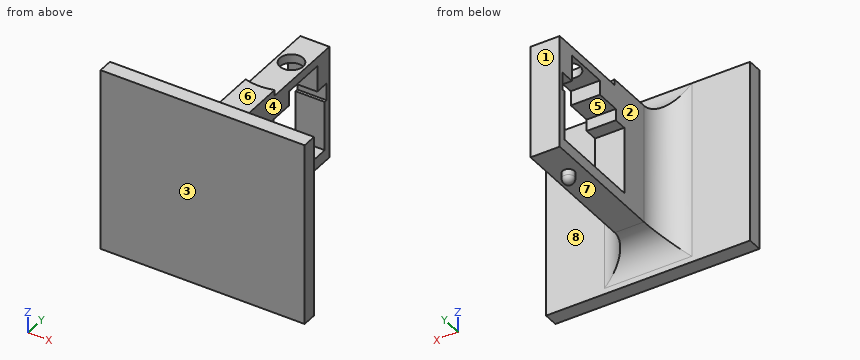
```python
from build123d import *

# Parameters (mm, degrees)
BOSS_EXTRUDE1_DEPTH      = 20
BOSS_EXTRUDE1_DEPTH_BACK = 43
SKETCH1_W                = 70
SKETCH1_H                = 5
BOSS_EXTRUDE2_DEPTH      = 10
BOSS_EXTRUDE2_DEPTH_BACK = 10
SKETCH2_W                = 10
SKETCH2_H                = 55
CUT_EXTRUDE2_DEPTH       = 10
CUT_EXTRUDE2_DEPTH_BACK  = 2
SKETCH4_R                = 1.25
SKETCH5_R                = 1.25
CUT_EXTRUDE3_DEPTH       = 20
CUT_EXTRUDE4_REACH       = 84.19
SKETCH6_W                = 3
SKETCH6_H                = 6
SKETCH6_H_2              = 17.5
SKETCH6_W_2              = 4
SKETCH6_H_3              = 5
SKETCH6_H_4              = 4.5
SKETCH6_W_3              = 5
SKETCH6_H_5              = 9
SKETCH6_W_4              = 13
SKETCH7_R                = 4
CUT_EXTRUDE5_DEPTH       = 6
SKETCH8_W                = 4
SKETCH8_H                = 15
SKETCH8_W_2              = 17
SKETCH8_H_2              = 20.5
BOSS_EXTRUDE3_DEPTH      = 10
SKETCH9_R                = 2
BOSS_EXTRUDE4_DEPTH      = 8
FILLET2_R                = 2
FILLET1_R                = 10


with BuildPart() as part:
    # Sketch1 → Boss-Extrude1 (new, two sides: drawn at the far end of the back side and taken through both)
    with BuildSketch(Plane.XY.offset(-BOSS_EXTRUDE1_DEPTH_BACK)):
        Rectangle(SKETCH1_W, SKETCH1_H)
    extrude(amount=BOSS_EXTRUDE1_DEPTH + BOSS_EXTRUDE1_DEPTH_BACK)

    # Sketch2 → Boss-Extrude2 (add, two sides: drawn at the far end of the back side and taken through both)
    with BuildSketch(Plane.XY.offset(-BOSS_EXTRUDE2_DEPTH_BACK)):
        with Locations((0, 30)):
            Rectangle(SKETCH2_W, SKETCH2_H)
    extrude(amount=BOSS_EXTRUDE2_DEPTH + BOSS_EXTRUDE2_DEPTH_BACK)

    # Sketch4 → Cut-Extrude2 (cut, two sides: drawn at the far end of the back side and taken through both)
    # profile 1 of 2: a face of its own
    with BuildSketch(Plane.XY.offset(10).offset(-CUT_EXTRUDE2_DEPTH_BACK)):
        with BuildLine():
            ThreePointArc((5, 28.229490169), (14.0312152, 34.541749668), (17.5, 45))
            ThreePointArc((17.5, 45), (-10.458250332, 59.0312152), (-5, 28.229490169))
            Line((-5, 28.229490169), (-5, 57.5))
            Line((-5, 57.5), (5, 57.5))
            Line((5, 57.5), (5, 28.229490169))
        make_face()
    # profile 2 of 2: a face of its own
    with BuildSketch(Plane.XY.offset(10).offset(-CUT_EXTRUDE2_DEPTH_BACK)):
        with BuildLine():
            Line((-5, 57.5), (-5, 28.229490169))
            ThreePointArc((-5, 28.229490169), (0, 27.5), (5, 28.229490169))
            Line((5, 28.229490169), (5, 57.5))
            Line((5, 57.5), (-5, 57.5))
        make_face()
        with Locations((0, 45)):
            Circle(SKETCH4_R, mode=Mode.SUBTRACT)
    extrude(amount=CUT_EXTRUDE2_DEPTH + CUT_EXTRUDE2_DEPTH_BACK, mode=Mode.SUBTRACT)

    # Sketch5 → Cut-Extrude3 (cut)
    with BuildSketch(Plane.XY.offset(10)):
        with Locations((0, 45)):
            Circle(SKETCH5_R)
    extrude(amount=-CUT_EXTRUDE3_DEPTH, mode=Mode.SUBTRACT)

    # Cut-Extrude4: up to this face of the body (flat: up to its plane)
    cut_extrude4_end = Plane(part.part.faces().sort_by_distance((5, 29.276865139, -0.505895275))[0])
    # Sketch6 → Cut-Extrude4 (cut, up to the picked face)
    with BuildSketch(Plane.ZY.offset(5), mode=Mode.PRIVATE) as cut_extrude4_sk1:
        with Locations((-5.5, 48)):
            Rectangle(SKETCH6_W, SKETCH6_H)
    cut_extrude4_tool1 = split(extrude(cut_extrude4_sk1.sketch, amount=-CUT_EXTRUDE4_REACH, mode=Mode.PRIVATE), bisect_by=cut_extrude4_end, keep=Keep.BOTH, mode=Mode.PRIVATE)
    # Sketch6 → Cut-Extrude4 (cut, up to the picked face)
    with BuildSketch(Plane.ZY.offset(5), mode=Mode.PRIVATE) as cut_extrude4_sk2:
        Polygon((-7, 27.5), (-7, 45), (-7, 51), (-23, 51), (-23, 27.5), (-10, 27.5), align=None)
    cut_extrude4_tool2 = split(extrude(cut_extrude4_sk2.sketch, amount=-CUT_EXTRUDE4_REACH, mode=Mode.PRIVATE), bisect_by=cut_extrude4_end, keep=Keep.BOTH, mode=Mode.PRIVATE)
    # Sketch6 → Cut-Extrude4 (cut, up to the picked face)
    with BuildSketch(Plane.ZY.offset(5), mode=Mode.PRIVATE) as cut_extrude4_sk3:
        with Locations((-5.5, 36.25)):
            Rectangle(SKETCH6_W, SKETCH6_H_2)
    cut_extrude4_tool3 = split(extrude(cut_extrude4_sk3.sketch, amount=-CUT_EXTRUDE4_REACH, mode=Mode.PRIVATE), bisect_by=cut_extrude4_end, keep=Keep.BOTH, mode=Mode.PRIVATE)
    # Sketch6 → Cut-Extrude4 (cut, up to the picked face)
    with BuildSketch(Plane.ZY.offset(5), mode=Mode.PRIVATE) as cut_extrude4_sk4:
        with Locations((-2, 48)):
            Rectangle(SKETCH6_W_2, SKETCH6_H)
    cut_extrude4_tool4 = split(extrude(cut_extrude4_sk4.sketch, amount=-CUT_EXTRUDE4_REACH, mode=Mode.PRIVATE), bisect_by=cut_extrude4_end, keep=Keep.BOTH, mode=Mode.PRIVATE)
    # Sketch6 → Cut-Extrude4 (cut, up to the picked face)
    with BuildSketch(Plane.ZY.offset(5), mode=Mode.PRIVATE) as cut_extrude4_sk5:
        Polygon((0, 45), (-4, 45), (-4, 27.5), (0, 27.5), (0, 36), align=None)
    cut_extrude4_tool5 = split(extrude(cut_extrude4_sk5.sketch, amount=-CUT_EXTRUDE4_REACH, mode=Mode.PRIVATE), bisect_by=cut_extrude4_end, keep=Keep.BOTH, mode=Mode.PRIVATE)
    # Sketch6 → Cut-Extrude4 (cut, up to the picked face)
    with BuildSketch(Plane.ZY.offset(5), mode=Mode.PRIVATE) as cut_extrude4_sk6:
        with Locations((-5.5, 53.5)):
            Rectangle(SKETCH6_W, SKETCH6_H_3)
    cut_extrude4_tool6 = split(extrude(cut_extrude4_sk6.sketch, amount=-CUT_EXTRUDE4_REACH, mode=Mode.PRIVATE), bisect_by=cut_extrude4_end, keep=Keep.BOTH, mode=Mode.PRIVATE)
    # Sketch6 → Cut-Extrude4 (cut, up to the picked face)
    with BuildSketch(Plane.ZY.offset(5), mode=Mode.PRIVATE) as cut_extrude4_sk7:
        Polygon((-23, 51), (-7, 51), (-7, 56), (-10, 56), (-23, 56), align=None)
    cut_extrude4_tool7 = split(extrude(cut_extrude4_sk7.sketch, amount=-CUT_EXTRUDE4_REACH, mode=Mode.PRIVATE), bisect_by=cut_extrude4_end, keep=Keep.BOTH, mode=Mode.PRIVATE)
    # Sketch6 → Cut-Extrude4 (cut, up to the picked face)
    with BuildSketch(Plane.ZY.offset(5), mode=Mode.PRIVATE) as cut_extrude4_sk8:
        with Locations((-8.5, 25.25)):
            Rectangle(SKETCH6_W, SKETCH6_H_4)
    cut_extrude4_tool8 = split(extrude(cut_extrude4_sk8.sketch, amount=-CUT_EXTRUDE4_REACH, mode=Mode.PRIVATE), bisect_by=cut_extrude4_end, keep=Keep.BOTH, mode=Mode.PRIVATE)
    # Sketch6 → Cut-Extrude4 (cut, up to the picked face)
    with BuildSketch(Plane.ZY.offset(5), mode=Mode.PRIVATE) as cut_extrude4_sk9:
        with Locations((-5.5, 25.25)):
            Rectangle(SKETCH6_W, SKETCH6_H_4)
    cut_extrude4_tool9 = split(extrude(cut_extrude4_sk9.sketch, amount=-CUT_EXTRUDE4_REACH, mode=Mode.PRIVATE), bisect_by=cut_extrude4_end, keep=Keep.BOTH, mode=Mode.PRIVATE)
    # Sketch6 → Cut-Extrude4 (cut, up to the picked face)
    with BuildSketch(Plane.ZY.offset(5), mode=Mode.PRIVATE) as cut_extrude4_sk10:
        with Locations((2.5, 48)):
            Rectangle(SKETCH6_W_3, SKETCH6_H)
    cut_extrude4_tool10 = split(extrude(cut_extrude4_sk10.sketch, amount=-CUT_EXTRUDE4_REACH, mode=Mode.PRIVATE), bisect_by=cut_extrude4_end, keep=Keep.BOTH, mode=Mode.PRIVATE)
    # Sketch6 → Cut-Extrude4 (cut, up to the picked face)
    with BuildSketch(Plane.ZY.offset(5), mode=Mode.PRIVATE) as cut_extrude4_sk11:
        with Locations((2.5, 40.5)):
            Rectangle(SKETCH6_W_3, SKETCH6_H_5)
    cut_extrude4_tool11 = split(extrude(cut_extrude4_sk11.sketch, amount=-CUT_EXTRUDE4_REACH, mode=Mode.PRIVATE), bisect_by=cut_extrude4_end, keep=Keep.BOTH, mode=Mode.PRIVATE)
    # Sketch6 → Cut-Extrude4 (cut, up to the picked face)
    with BuildSketch(Plane.ZY.offset(5), mode=Mode.PRIVATE) as cut_extrude4_sk12:
        with Locations((-16.5, 25.25)):
            Rectangle(SKETCH6_W_4, SKETCH6_H_4)
    cut_extrude4_tool12 = split(extrude(cut_extrude4_sk12.sketch, amount=-CUT_EXTRUDE4_REACH, mode=Mode.PRIVATE), bisect_by=cut_extrude4_end, keep=Keep.BOTH, mode=Mode.PRIVATE)
    add(cut_extrude4_tool1.solids().sort_by(Axis((-5, 48, -5.5), (1, 0, 0)))[0], mode=Mode.SUBTRACT)
    add(cut_extrude4_tool2.solids().sort_by(Axis((-5, 39.25, -15), (1, 0, 0)))[0], mode=Mode.SUBTRACT)
    add(cut_extrude4_tool3.solids().sort_by(Axis((-5, 36.25, -5.5), (1, 0, 0)))[0], mode=Mode.SUBTRACT)
    add(cut_extrude4_tool4.solids().sort_by(Axis((-5, 48, -2), (1, 0, 0)))[0], mode=Mode.SUBTRACT)
    add(cut_extrude4_tool5.solids().sort_by(Axis((-5, 36.25, -2), (1, 0, 0)))[0], mode=Mode.SUBTRACT)
    add(cut_extrude4_tool6.solids().sort_by(Axis((-5, 53.5, -5.5), (1, 0, 0)))[0], mode=Mode.SUBTRACT)
    add(cut_extrude4_tool7.solids().sort_by(Axis((-5, 53.5, -15), (1, 0, 0)))[0], mode=Mode.SUBTRACT)
    add(cut_extrude4_tool8.solids().sort_by(Axis((-5, 25.25, -8.5), (1, 0, 0)))[0], mode=Mode.SUBTRACT)
    add(cut_extrude4_tool9.solids().sort_by(Axis((-5, 25.25, -5.5), (1, 0, 0)))[0], mode=Mode.SUBTRACT)
    add(cut_extrude4_tool10.solids().sort_by(Axis((-5, 48, 2.5), (1, 0, 0)))[0], mode=Mode.SUBTRACT)
    add(cut_extrude4_tool11.solids().sort_by(Axis((-5, 40.5, 2.5), (1, 0, 0)))[0], mode=Mode.SUBTRACT)
    add(cut_extrude4_tool12.solids().sort_by(Axis((-5, 25.25, -16.5), (1, 0, 0)))[0], mode=Mode.SUBTRACT)

    # Sketch7 → Cut-Extrude5 (cut)
    with BuildSketch(Plane(origin=(0, 0, 5), x_dir=(-1, 0, 0), z_dir=(0, 0, -1))):
        with Locations(Location((0, 45, 0), (0, 0, 90))):
            Circle(SKETCH7_R)
    extrude(amount=-CUT_EXTRUDE5_DEPTH, mode=Mode.SUBTRACT)

    # Sketch8 → Boss-Extrude3 (add)
    with BuildSketch(Plane.ZY.offset(5)):
        Polygon((-10, 55), (-10, 57.5), (-31, 57.5), (-31, 55), (-27, 55), align=None)
        with Locations((-29, 47.5)):
            Rectangle(SKETCH8_W, SKETCH8_H)
        Polygon((-27, 40), (-31, 40), (-31, 2.5), (-27, 2.5), (-27, 23), align=None)
        with Locations((-18.5, 12.75)):
            Rectangle(SKETCH8_W_2, SKETCH8_H_2)
    extrude(amount=-BOSS_EXTRUDE3_DEPTH)

    # Sketch9 → Boss-Extrude4 (add)
    with BuildSketch(Plane.XY.offset(-27)):
        with Locations((0, 45)):
            Circle(SKETCH9_R)
    extrude(amount=-BOSS_EXTRUDE4_DEPTH)

    # Fillet2
    fillet2_edges = [part.edges().sort_by_distance(p)[0] for p in [
        (-2, 45, -35),
    ]]
    fillet(fillet2_edges, radius=FILLET2_R)

    # Fillet1
    fillet1_edges = [part.edges().sort_by_distance(p)[0] for p in [
        (0, 2.5, -31),
        (5, 2.5, -10.5),
        (-5, 2.5, -10.5),
        (0, 2.5, 10),
    ]]
    fillet(fillet1_edges, radius=FILLET1_R - 0.0001)  # a hair under: the kernel refuses the full size


solid = part.part
```
Here's how the part is built. I have some questions about the finished solid (model axes, mm). Face numbers are marked on the shaded views. A direction names the side the tool comes from. Coordinates: 2 decimals unless noted, no trailing zeros. Order: outer loops, then holes, each group sorted by start corner. A loop starts at its lowest first (then second) coordinate and runs counter-clockwise, first axis right, second up. Notation, with made-up numbers: M -26.75,20 L 26.25,20 A25 ccw 26.25,38 Z; hole C -3,48 d4. An arc over 180 degrees is marked long. Answer as a JSON object with one key per item and string values. Group by question number.
(1) I need wall thicknesses on probe 1 along Z at (x, y) = (0.5, 30); probe 2 along X at (y, z) = (45, 5.85); probe 3 along X at (y, z) = (16, -28). Which ranges of each line are inside material? Lowest first, please.
(2) Suppose I cut it at A-A, the plane y = 38.5. Please give me the cut outline in (x, z).
(3) Suppose I cut it at B-B, the plane z = 3.5. Please give me the cut outline in (x, y), then the cut area to 3 significant figures.
(4) If we mould it in two halves opening along Y, with no side actions, what happens to the marked faces 6, 7 and 8? For each: released by +Y, released by -Y, zero draft, split by the parting line, or undercut.
(5) For pin 1 (6 mm diameter, centred on x = 9, y = 31.5, fed in from +Z); pin 2 (9 mm diameter, centred on x = 0, y = 45, fed in from +Z); pin 3 (5 mm diameter, centred on y = 18.5, z = 1, fed in from +X); pin 4 (4 mm diameter, centred on x = 16, z = -0.5, fed in from +Y), each with a flat end and sliding along its axis, tell me the tip position at first contact or that it passes through.
(6) Which directions (+Z, -Z, +X, -X, +Y, -Y) give clear straight access to the entire face, cutting with the end or side of a thin tool? Please do the marked faces 1, 2, 3, 4 and 5.
(7) Suppose I cut it at C-C, the plane y = 45. Please give me the cut outline in (x, z).
Values found:
{
 "1": {"probe 1": "z = -31 to -27, 0 to 8", "probe 2": "x = -5 to -4, 4 to 5", "probe 3": "x = -5 to 5"},
 "2": {"outline": "M -5,-31 L 5,-31 L 5,-27 L -5,-27 Z; M -5,5 L 5,5 L 5,8 L -5,8 Z"},
 "3": {"outline": "M -35,-2.5 L 35,-2.5 L 35,2.5 L 15,2.5 A10 cw 5,12.5 L 5,36 L -5,36 L -5,12.5 A10 cw -15,2.5 L -35,2.5 Z; M -5,51 L 5,51 L 5,57.5 L -5,57.5 Z", "area": "793 mm^2"},
 "4": {"face 6": "zero draft", "face 7": "undercut", "face 8": "released by +Y"},
 "5": {"pin 1": "passes through", "pin 2": "stops at z = 8", "pin 3": "stops at x = 5", "pin 4": "stops at y = 2.55"},
 "6": {"face 1": "+Z, -Z, +X, -X, +Y", "face 2": "+Z, -Z, -X, +Y", "face 3": "+Z, -Z, +X, -X, -Y", "face 4": "+Z, -Z, +X, +Y", "face 5": "+X, -X"},
 "7": {"outline": "M -5,-31 L -2,-31 L -2,-33 A2 ccw 2,-33 L 2,-31 L 5,-31 L 5,-27 L -5,-27 Z; M -5,5 L -4,5 L -4,8 L -5,8 Z; M 4,5 L 5,5 L 5,8 L 4,8 Z"}
}
